The figure shows three views and two pictorial views of one solid part (mm, origin at its lowest corner). Answer the questions. Round coordinates to 2 decimals unless told otherwise and drop trailing zeros. Order: outer loops, then holes, each group sorted by start corner. A loop starts at its lowest first (then second) coordinate and runs counter-clockwise, first axis right, second up. Notation, with made-up numbers: M 2,54.25 L 6,54.25 A23 cw 6,70.25 Z; hole C -21.5,4.25 d5. An arc over 180 degrees is marked long. Return JSON: item names as keys, results as strings.
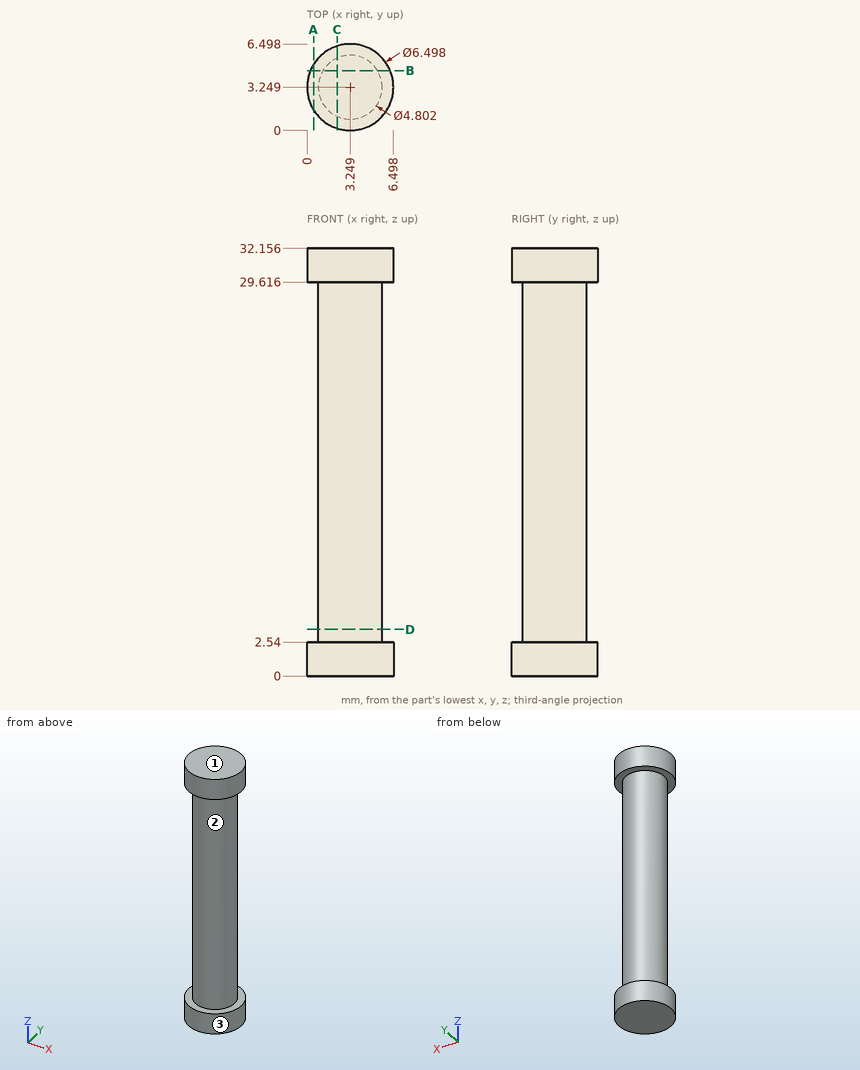
Item 1: Find section D-D (z = 3.5). Determine the outline of the cut face in (x, y).
Output:
{"outline": "C 3.25,3.25 d4.8"}
Item 2: Each of these flat-tipped pins is pushed along its axis until it touches: pin 1 (1.5 mm diameter, centred on x = 1.5, z = 28, fed in from -Y) (1 decimal); pin 2 (1.5 mm diameter, centred on x = 1, z = 14, fed in from -Y). Where does it stop, or does it pass through?
Output:
{"pin 1": "stops at y = 1.1", "pin 2": "stops at y = 1.37"}
Item 3: Consider line 1 along Z through (x, y) = (4.75, 0.5); line 2 along Y through (x, z) = (6, 30) (1 decimal); line 3 along Y through (x, z) = (2, 16). Determine where each line is inside the solid, lowest interval first. Write a range as [from, to].
Output:
{"line 1": "z = [0, 2.54], [29.62, 32.16]", "line 2": "y = [1.5, 5]", "line 3": "y = [1.2, 5.3]"}
Item 4: Find section B-B (y = 4.5). Determine the outline of the cut face in (x, z).
Output:
{"outline": "M 0.25,0 L 6.25,0 L 6.25,2.54 L 5.3,2.54 L 5.3,29.62 L 6.25,29.62 L 6.25,32.16 L 0.25,32.16 L 0.25,29.62 L 1.2,29.62 L 1.2,2.54 L 0.25,2.54 Z"}
Item 5: Find section C-C (x = 2.25). Determine the outline of the cut face in (y, z) (1 decimal).
Output:
{"outline": "M 0.2,0 L 6.3,0 L 6.3,2.5 L 5.4,2.5 L 5.4,29.6 L 6.3,29.6 L 6.3,32.2 L 0.2,32.2 L 0.2,29.6 L 1.1,29.6 L 1.1,2.5 L 0.2,2.5 Z"}
Item 6: Find section A-A (x = 0.5). Determine the outline of the cut face in (y, z), plus the area to 3 significant figures.
Output:
{"outline": "M 1.52,0 L 4.98,0 L 4.98,2.54 L 1.52,2.54 Z; M 1.52,29.62 L 4.98,29.62 L 4.98,32.16 L 1.52,32.16 Z", "area": "17.6 mm^2"}
Item 7: The mould has two halves that part along Z. Classify the marked faces 1, 2 and 3: pulls with the +Z half, pulls with the -Z half, needs draft (parallel to the pull), parting line crosses it, or undercut.
Output:
{"face 1": "pulls with the +Z half", "face 2": "undercut", "face 3": "needs draft"}
